Input: part model. Units: mm. Frame: model coordinates. Face numbers are marked on the shaded views. A direction names the side the tool comes from. Round coordinates to 2 decimals unless told otherwise and drop trailing zeros. Loops run counter-clockwise (first coordinate to the right, second up) from the corner with the lowest first, then second, coordinate; pieces in that order, holes last. Notation, with made-up numbers: (-25, -11.5) - (-13, -11.5) arc R23 ccw to (-13, 9.5) - close; hole circle Ø8 at (77, 48.25). An arc over 180 degrees is marked (long way). Write each question's results on one line, items separated by ' | '.
from build123d import *

# Parameters (mm, degrees)
SKETCH1_W           = 35
SKETCH1_H           = 40
BOSS_EXTRUDE1_DEPTH = 40
SKETCH2_W           = 10
SKETCH2_H           = 10
CUT_EXTRUDE1_DEPTH  = 15
SKETCH3_W           = 10
SKETCH3_H           = 10
CUT_EXTRUDE2_DEPTH  = 5
SKETCH4_W           = 25
SKETCH4_H           = 30
CUT_EXTRUDE3_DEPTH  = 10
CUT_EXTRUDE4_DEPTH  = 31
CUT_EXTRUDE5_DEPTH  = 10
CUT_EXTRUDE6_DEPTH  = 20
CUT_EXTRUDE7_DEPTH  = 20


with BuildPart() as part:
    # Sketch1 → Boss-Extrude1 (new body)
    with BuildSketch(Plane.XY):
        Rectangle(SKETCH1_W, SKETCH1_H)
    extrude(amount=BOSS_EXTRUDE1_DEPTH)

    # Sketch2 → Cut-Extrude1 (cut)
    with BuildSketch(Plane.XY.offset(40)):
        with Locations((12.5, 15)):
            Rectangle(SKETCH2_W, SKETCH2_H)
    extrude(amount=-CUT_EXTRUDE1_DEPTH, mode=Mode.SUBTRACT)

    # Sketch3 → Cut-Extrude2 (cut)
    with BuildSketch(Plane.XY.offset(40)):
        with Locations((-12.5, -15)):
            Rectangle(SKETCH3_W, SKETCH3_H)
    extrude(amount=-CUT_EXTRUDE2_DEPTH, mode=Mode.SUBTRACT)

    # Sketch4 → Cut-Extrude3 (cut)
    with BuildSketch(Plane.XY.offset(40)):
        with Locations((-5, 5)):
            Rectangle(SKETCH4_W, SKETCH4_H)
    extrude(amount=-CUT_EXTRUDE3_DEPTH, mode=Mode.SUBTRACT)

    # Sketch5 → Cut-Extrude4 (cut, through all)
    with BuildSketch(Plane.XY.offset(30)):
        Polygon((2.5, 20), (-17.5, -20), (-17.5, 20), align=None)
    extrude(amount=-CUT_EXTRUDE4_DEPTH, mode=Mode.SUBTRACT)

    # Sketch6 → Cut-Extrude5 (cut)
    with BuildSketch(Plane.XY.offset(35)):
        Polygon((-12.5, -10), (-17.5, -20), (-17.5, -10), align=None)
    extrude(amount=-CUT_EXTRUDE5_DEPTH, mode=Mode.SUBTRACT)

    # Sketch7 → Cut-Extrude6 (cut)
    with BuildSketch(Plane.XY.offset(30)):
        Polygon((7.5, 20), (2.5, 20), (-2.5, 10), (7.5, 10), align=None)
    extrude(amount=-CUT_EXTRUDE6_DEPTH, mode=Mode.SUBTRACT)

    # Sketch13 → Cut-Extrude7 (cut)
    with BuildSketch(Plane(origin=(0, 10, 10), x_dir=(1, 0, 0), z_dir=(0, 0.707106781, 0.707106781))):
        Polygon((7.5, 0), (7.5, -28.284271247), (-12.5, -28.284271247), (-2.5, 0), align=None)
    extrude(amount=CUT_EXTRUDE7_DEPTH, mode=Mode.SUBTRACT)


solid = part.part
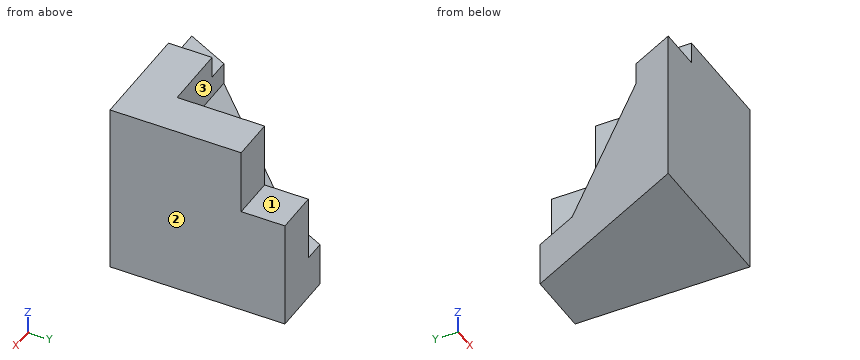
1. Contact query for flat-ended pins moving along their axis: pin 1 (3 mm diameter, centred on x = -5.5, z = 35.5, fed in from +Y); pin 2 (8 mm diameter, centred on x = 4, y = 17, fed in from +Z); pin 3 (2.5 mm diameter, centred on y = -17, z = 38, fed in from -X); pin 4 (8 mm diameter, centred on x = 15, y = 13.5, fed in from +Z). Output: stop coordinate, or through.
Answer:
pin 1: y = -10 | pin 2: z = 25 | pin 3: x = -7.5 | pin 4: z = 40
2. Section query B-B, the plane z = 15. Output: boundary loops of the cut face in (x, y), plus the area to 3 significant figures.
Answer:
outline: (-17.5, -20) - (17.5, -20) - (17.5, 20) - (7.5, 20) - (7.5, 5) - (-5, 5) - close | area: 869 mm^2
3. Line query: line 1 (Z direction, x = 9.5, y = 14); line 2 (Y direction, x = 12, z = 27.5); line 3 (X direction, y = 10.5, z = 13). Output: solid intervals per line, ascending. Write a range as [from, to].
Answer:
line 1: [0, 25] | line 2: [-20, 10] | line 3: [7.5, 17.5]
4. Set-up query: the marked faces 1, 2 and 3. Return all of +Z, -Z, +X, -X, +Y, -Y with unobstructed straight access to the full face (end or side cutting, diameter ignored); none if empty.
Answer:
face 1: +Z, +X, -X, +Y | face 2: +Z, -Z, +X, +Y, -Y | face 3: +Z, -X, +Y
5. Section query C-C, the plane y = -2.5. Output: boundary loops of the cut face in (x, z).
Answer:
outline: (-8.75, 0) - (17.5, 0) - (17.5, 40) - (7.5, 40) - (7.5, 22.5) - (-8.75, 22.5) - close
6. Section query D-D, the plane z = 7.5. Output: boundary loops of the cut face in (x, y), plus the area to 3 significant figures.
Answer:
outline: (-17.5, -20) - (17.5, -20) - (17.5, 20) - (2.5, 20) - close | area: 1,000 mm^2
7. Section query A-A, the plane x = 1.5. Output: boundary loops of the cut face in (y, z), plus the area to 3 significant figures.
Answer:
outline: (-20, 0) - (18, 0) - (18, 10) - (10, 10) - (-10, 30) - (-10, 40) - (-20, 40) - close | area: 880 mm^2
